The listing builds one solid part. Answer for the finished solid, in the listing's coordinates (mm). A direction names the side the tool comes from. Round coordinates to 2 decimals unless told otherwise and drop trailing zeros. Write each loop counter-clockwise with the first axis right and the second up, starting at its lowest first coordinate (ties: lowest second). Pieces come first, ordered by that corner, then holes. Notation, with made-up numbers: M 67,70.5 L 76,70.5 A27 cw 76,97.5 Z; hole C 30,45.25 d11. An arc over 180 degrees is marked long. One line per item, written item: value. Start each with the question number.
(1) Section A-A (z = -7.75) is taken. Determine the outline of the cut face in (x, y).
(2) Given P1, Ø6, axis at y = -1, z = -9.5, coming from the +X side; P2, Ø6, axis at x = -31, z = -4, coming from the -Y side; P3, Ø7, axis at y = -4.79, z = -12.22, coming from the -X side, each flat-ended and moving along its own axis, determine where each tip first touches the part or whether it passes through.
(3) Section C-C (z = -10.75) is taken. Determine the outline of the cut face in (x, y), plus the area to 3 significant figures.
(4) Section B-B (y = 2) is taken. State how many separate pieces and enclosed holes the cut face has, plus the area to 3 significant figures.
(5) For faces 4 (the cylindrical face through (1.701, -2.558, -11.931)), 5 (the flat face through (0.463, -2, -3)), determine the directions among +Z, -Z, +X, -X, +Y, -Y from which every point of the face is accessible in a straight line to the end or side of a thin tool.
(6) For a pull along Y with two mould halves and no side action, classify faces 1 (the cylindrical face through (1.7, 3.9, -14.37)), 2 (the flat face through (-24, -13.015, -2)), 3 (the flat face through (2, -1, -15.77)) as released by +Y, released by -Y, zero draft, split by the parting line, or undercut.
(7) Consider probe 1 along X at (y, z) = (-10, -14.5); probe 2 along Z at (x, y) = (-20, -1.25). Determine where each line is inside the solid, lowest interval first.
```python
from build123d import *

# Parameters (mm, degrees)
BOSS_EXTRUDE3_DEPTH       = 10
BOSS_EXTRUDE3_DEPTH_BACK  = 13.014944575
SKETCH1_W                 = 53
SKETCH1_H                 = 2
SKETCH2_W                 = 2.504977783
SKETCH2_H                 = 23.010208786
BOSS_EXTRUDE4_DEPTH       = 12
SKETCH3_W                 = 2.506556419
SKETCH3_H                 = 23.01450768
BOSS_EXTRUDE5_DEPTH       = 11.990007083
BOSS_EXTRUDE6_START       = -52.981944033
BOSS_EXTRUDE6_OUTLINE_R   = 2.248774255
BOSS_EXTRUDE6_OUTLINE_R_2 = 2.25
BOSS_EXTRUDE6_DEPTH       = 52.981944033
SKETCH6_W                 = 47.946959802
SKETCH6_H                 = 0.996975491
CUT_EXTRUDE2_DEPTH        = 29


# Read off the part's stored shape, not the designer's step: Boss-Extrude6
with BuildPart() as part:
    # Sketch1 → Boss-Extrude3 (new, two sides: drawn at the far end of the back side and taken through both)
    with BuildSketch(Plane(origin=(0, 0, 0), x_dir=(1, 0, 0), z_dir=(0, 1, 0)).offset(-BOSS_EXTRUDE3_DEPTH_BACK)):
        with Locations((-23.514130948, 2.769901189)):
            Rectangle(SKETCH1_W, SKETCH1_H)
    extrude(amount=BOSS_EXTRUDE3_DEPTH + BOSS_EXTRUDE3_DEPTH_BACK)

    # Sketch2 → Boss-Extrude4 (add)
    with BuildSketch(Plane(origin=(-2.522360337, 0, -3.769901189), x_dir=(-1, 0, 0), z_dir=(0, 0, -1))):
        with Locations((-4.240718342, -1.512860106)):
            Rectangle(SKETCH2_W, SKETCH2_H)
    extrude(amount=BOSS_EXTRUDE4_DEPTH)

    # Sketch3 → Boss-Extrude5 (add)
    with BuildSketch(Plane(origin=(0, 0, -3.769901189), x_dir=(-1, 0, 0), z_dir=(0, 0, -1))):
        with Locations((48.757818929, -1.500170116)):
            Rectangle(SKETCH3_W, SKETCH3_H)
    extrude(amount=BOSS_EXTRUDE5_DEPTH)

    # Boss-Extrude6 outline → Boss-Extrude6 (cut)
    with BuildSketch(Plane(origin=(2.970846895, 0, 0), x_dir=(0, 0, -1), z_dir=(1, 0, 0)).offset(BOSS_EXTRUDE6_START)):
        with Locations((12.226476123, 3.226243709)):
            Circle(BOSS_EXTRUDE6_OUTLINE_R)
        with Locations((12.224283194, -4.788420336)):
            Circle(BOSS_EXTRUDE6_OUTLINE_R_2)
    extrude(amount=BOSS_EXTRUDE6_DEPTH, mode=Mode.SUBTRACT)

    # Sketch6 → Cut-Extrude2 (cut)
    with BuildSketch(Plane(origin=(0, -13.014944575, 0), x_dir=(-1, 0, 0), z_dir=(0, -1, 0))):
        with Locations((23.509982369, 3.279148845)):
            Rectangle(SKETCH6_W, SKETCH6_H)
    extrude(amount=-CUT_EXTRUDE2_DEPTH, mode=Mode.SUBTRACT)


solid = part.part
```
Recorded:
1. outline: M -50.01,-13.01 L -47.5,-13.01 L -47.5,10.01 L -50.01,10.01 Z; M 0.47,-13.02 L 2.97,-13.02 L 2.97,9.99 L 0.47,9.99 Z
2. P1: stops at x = 2.97
2. P2: stops at y = -13.01
2. P3: stops at x = -50.01
3. outline: M -50.01,-13.01 L -47.5,-13.01 L -47.5,-6.49 L -50.01,-6.49 Z; M -50.01,-3.09 L -47.5,-3.09 L -47.5,1.53 L -50.01,1.53 Z; M -50.01,4.92 L -47.5,4.92 L -47.5,10.01 L -50.01,10.01 Z; M 0.47,-13.02 L 2.97,-13.02 L 2.97,-6.49 L 0.47,-6.49 Z; M 0.47,-3.09 L 2.97,-3.09 L 2.97,1.53 L 0.47,1.53 Z; M 0.47,4.92 L 2.97,4.92 L 2.97,9.99 L 0.47,9.99 Z
3. area: 81.3 mm2
4. separate pieces: 3
4. enclosed holes: 0
4. area: 99.8 mm2
5. face 4: +X, -X
5. face 5: -Z, +Y, -Y
6. face 1: undercut
6. face 2: released by -Y
6. face 3: zero draft
7. probe 1: x = -50.01 to -47.5, 0.47 to 2.97
7. probe 2: z = -2.78 to -1.77
